from build123d import *

# Parameters (mm, degrees)
SKETCH1_R                = 14.5
BOSS_EXTRUDE1_DEPTH      = 3
M4_CLEARANCE_HOLE1_D     = 4
M4_CLEARANCE_HOLE1_DEPTH = 10
M4_CLEARANCE_HOLE1_TIP   = 1.201721238
CIRPATTERN1_COUNT        = 6
M4_CLEARANCE_HOLE3_D     = 4


with BuildPart() as part:
    # Sketch1 → Boss-Extrude1 (new body)
    with BuildSketch(Plane.XY):
        with BuildLine():
            Line((-125, 10.558810184), (-125, -86.112499703))
            ThreePointArc((-125, -86.112499703), (-123.915997441, -89.221352232), (-121.134014383, -90.982203121))
            Line((-121.134014383, -90.982203121), (-9.639122255, -116.946168572))
            ThreePointArc((-9.639122255, -116.946168572), (0, -118.053689519), (9.639122255, -116.946168572))
            Line((9.639122255, -116.946168572), (121.134014383, -90.982203121))
            ThreePointArc((121.134014383, -90.982203121), (123.915997441, -89.221352232), (125, -86.112499703))
            Line((125, -86.112499703), (125, 10.558810184))
            ThreePointArc((125, 10.558810184), (123.768755522, 13.844610211), (120.681407274, 15.512160982))
            Line((120.681407274, 15.512160982), (53.407036368, 24.76675399))
            ThreePointArc((53.407036368, 24.76675399), (40.948782136, 23.303979385), (30.769230769, 15.974276659))
            ThreePointArc((30.769230769, 15.974276659), (0, 1.533119315), (-30.769230769, 15.974276659))
            ThreePointArc((-30.769230769, 15.974276659), (-40.948782136, 23.303979385), (-53.407036368, 24.76675399))
            Line((-53.407036368, 24.76675399), (-120.681407274, 15.512160982))
            ThreePointArc((-120.681407274, 15.512160982), (-123.768755522, 13.844610211), (-125, 10.558810184))
        make_face()
        with Locations((0, -75.553689519)):
            Circle(SKETCH1_R, mode=Mode.SUBTRACT)
    extrude(amount=BOSS_EXTRUDE1_DEPTH)

    # M4 Clearance Hole1
    with Locations(Plane.XY.offset(3)):
        with Locations((-66, 0), (-34, 0), (-50, 16), (-50, -16), (34, 0), (50, 16), (66, 0), (50, -16)):
            Hole(M4_CLEARANCE_HOLE1_D / 2, depth=M4_CLEARANCE_HOLE1_DEPTH)
            with Locations((0, 0, -(M4_CLEARANCE_HOLE1_DEPTH + M4_CLEARANCE_HOLE1_TIP / 2))):  # 118° drill point
                Cone(0, M4_CLEARANCE_HOLE1_D / 2, M4_CLEARANCE_HOLE1_TIP, mode=Mode.SUBTRACT)

    # Sketch8 → M4 Clearance Hole2 (revolve, cut)
    with BuildSketch(Plane(origin=(0, -108.053689519, 3), x_dir=(0, -1, 0), z_dir=(1, 0, 0))):
        Polygon((0, 0), (0, 11.201721238), (2, 10), (2, 0), align=None)
    m4_clearance_hole2 = revolve(axis=Axis((0, -108.053689519, 9.35), (0, 0, -1)), mode=Mode.SUBTRACT)

    # CirPattern1: M4 Clearance Hole2 ×6 about axis
    cirpattern1_axis = Axis((0, -75.553689519, 0), (0, 0, 1))
    for i in range(1, CIRPATTERN1_COUNT):
        add(m4_clearance_hole2.rotate(cirpattern1_axis, i * 360 / CIRPATTERN1_COUNT), mode=Mode.SUBTRACT)

    # M4 Clearance Hole3 (through all)
    with Locations(Plane.XY.offset(3)):
        with Locations((-120, 10.558810184), (-107, 10.558810184), (-120, -31.441189816), (-107, -31.441189816), (-120, -86.112499703), (-107, -44.112499703), (-120, -44.112499703), (-107, -86.112499703), (120, 10.558810184), (107, -31.441189816), (120, -31.441189816), (107, 10.558810184), (120, -86.112499703), (107, -44.112499703), (120, -44.112499703), (107, -86.112499703)):
            Hole(M4_CLEARANCE_HOLE3_D / 2)


solid = part.part
CAD build for the part. Positions are in the model's coordinates, mm. Give positions to 0.01 mm unless a question says otherwise; leave off trailing zeros. Write each loop counter-clockwise with the first axis right and the second up, starting at its lowest first coordinate (ties: lowest second). Pieces come first, ordered by that corner, then holes. Notation, with made-up numbers: (29.5, -39) -> (82.5, -39) arc R32 cw to (82.5, -2) -> close; hole circle Ø7 at (86.25, -27.75). An arc over 180 degrees is marked (long way). Return JSON: item names as keys, results as strings.
Item 1: Drill centre lines: probe 1 along Y at (x, z) = (-120, 1); probe 2 along Y at (x, z) = (-51.5, 1.1); probe 3 along X at (y, z) = (15, 2.8). Where is each one in solid material? Low to high.
Answer below:
{"probe 1": "y = -91.25 to -88.11, -84.11 to -46.11, -42.11 to -33.44, -29.44 to 8.56, 12.56 to 15.61", "probe 2": "y = -107.2 to -17.32, -14.68 to 14.68, 17.32 to 24.95", "probe 3": "x = -122.3 to -51.73, -48.27 to -29.93, 29.93 to 48.27, 51.73 to 122.3"}
Item 2: Two-plate mould, pull along X, no slides. Class faces 1 (the cylindrical face through (41.114, 23.368, 1.479)), 2 (the flat face through (-2, -46, 0)), 3 (the flat face through (87.515, 20.075, 1.479)): +X half, -X half, draft (parallel to the pull), parting line (faces both ways), or undercut.
Answer below:
{"face 1": "undercut", "face 2": "draft", "face 3": "+X half"}
Item 3: Drop a flat-ended pin along its axis: pin 1 (1 mm diameter, centred on x = -86, z = 0.5, fed in from -Y). Give the stop position or say it passes through.
Answer below:
{"pin 1": "stops at y = -99.28"}
Item 4: Band-saw the part on C-C (x = -80.5). List the corners of the cut face in (y, z), then the cut area to 3 significant figures.
Answer below:
{"outline": "(-100.44, 0) -> (21.04, 0) -> (21.04, 3) -> (-100.44, 3) -> close", "area": "364 mm2"}
Item 5: Band-saw the part on A-A (z = 1.4). Give the number of separate pieces and of enclosed holes in the cut face, then the cut area to 3 significant figures.
Answer below:
{"separate pieces": "1", "enclosed holes": "31", "area": "29,300 mm2"}
Item 6: Band-saw the part on B-B (x = 58). List the corners of the cut face in (y, z).
Answer below:
{"outline": "(-105.68, 0) -> (24.13, 0) -> (24.13, 3) -> (-105.68, 3) -> close"}
